Could you check a few things on this model? Use its own coordinates, in mm. Give positions to 0.01 mm unless a question says otherwise; leave off trailing zeros. Write each question's results on one line, items separated by ' | '. Start each with the question number.
Q1. Will this pin go through, and if not, where does the flat tip stop? P1, Ø1.5, axis at y = -1, z = -189, coming from the +X side.
Q2. If I drill on line 1 along X through (y, z) = (0.6, -190); line 2 along Z through (x, y) = (130, -0.45); line 3 along Z through (x, y) = (210, -0.75), over which ranges is the centre line in solid material (lowest first)?
Q3. If we section it at A-A, the plane y = 0.75: Give the number of separate pieces and of enclosed holes in the cut face, plus the area to 3 significant figures.
from build123d import *

# Parameters (mm, degrees)
SKETCH1_W               = 440
SKETCH1_H               = 400
BOSS_EXTRUDE1_DEPTH     = 2.5
SKETCH2_W               = 22
SKETCH2_H               = 22
CUT_EXTRUDE1_DEPTH      = 5
SKETCH3_R               = 2.6
CUT_EXTRUDE2_DEPTH      = 5
MIRROR2_COPY_1_SKETCH_W = 22
MIRROR2_COPY_1_SKETCH_H = 22
MIRROR2_COPY_1_DEPTH    = 5
MIRROR2_COPY_2_SKETCH_R = 2.6
MIRROR2_COPY_2_DEPTH    = 5
FILLET1_R               = 5
SKETCH4_W               = 25
SKETCH4_H               = 5
CUT_EXTRUDE3_DEPTH      = 5
LPATTERN1_COUNT         = 8
LPATTERN1_PITCH         = 55
SKETCH5_R               = 2.6
CUT_EXTRUDE4_DEPTH      = 5
LPATTERN2_COUNT         = 7
LPATTERN2_PITCH         = 55
SKETCH6_W               = 42.3
SKETCH6_H               = 42.3
CUT_EXTRUDE5_DEPTH      = 5
FILLET2_R               = 4
SKETCH7_R               = 2.6
CUT_EXTRUDE7_DEPTH      = 5
LPATTERN3_COUNT         = 2
LPATTERN3_PITCH         = 60
LPATTERN3_COUNT_DIR2    = 2
LPATTERN3_PITCH_DIR2    = 30
SKETCH8_R               = 4
SKETCH8_R_2             = 2.6
CUT_EXTRUDE8_DEPTH      = 5
CUT_EXTRUDE9_DEPTH      = 5


with BuildPart() as part:
    # Sketch1 → Boss-Extrude1 (new, symmetric)
    with BuildSketch(Plane(origin=(0, 0, 0), x_dir=(1, 0, 0), z_dir=(0, 1, 0))):
        Rectangle(SKETCH1_W, SKETCH1_H)
    extrude(amount=BOSS_EXTRUDE1_DEPTH, both=True)

    # Sketch2 → Cut-Extrude1 (cut)
    with BuildSketch(Plane(origin=(0, 2.5, 0), x_dir=(1, 0, 0), z_dir=(0, 1, 0))):
        with Locations((209, 189)):
            Rectangle(SKETCH2_W, SKETCH2_H)
    cut_extrude1 = extrude(amount=-CUT_EXTRUDE1_DEPTH, mode=Mode.SUBTRACT)

    # Sketch3 → Cut-Extrude2 (cut)
    with BuildSketch(Plane(origin=(0, 2.5, 0), x_dir=(1, 0, 0), z_dir=(0, 1, 0))):
        with Locations(Location((190, 190, 0), (0, 0, 270))):
            Circle(SKETCH3_R)
        with Locations(Location((210, 170, 0), (0, 0, 270))):
            Circle(SKETCH3_R)
    cut_extrude2 = extrude(amount=-CUT_EXTRUDE2_DEPTH, mode=Mode.SUBTRACT)

    # Mirror1: Cut-Extrude1, Cut-Extrude2 across plane
    add(cut_extrude1.mirror(Plane(origin=(0, 0, 0), x_dir=(0, 0, 1), z_dir=(1, 0, 0))), mode=Mode.SUBTRACT)
    add(cut_extrude2.mirror(Plane(origin=(0, 0, 0), x_dir=(0, 0, 1), z_dir=(1, 0, 0))), mode=Mode.SUBTRACT)

    # Mirror2: Cut-Extrude1, Cut-Extrude2 across plane
    add(cut_extrude1.mirror(Plane.XY), mode=Mode.SUBTRACT)
    add(cut_extrude2.mirror(Plane.XY), mode=Mode.SUBTRACT)

    # Mirror2 copy 1 sketch → Mirror2 copy 1 (cut)
    with BuildSketch(Plane(origin=(0, 2.5, 0), x_dir=(-1, 0, 0), z_dir=(0, 1, 0))):
        with Locations((209, 189)):
            Rectangle(MIRROR2_COPY_1_SKETCH_W, MIRROR2_COPY_1_SKETCH_H)
    extrude(amount=-MIRROR2_COPY_1_DEPTH, mode=Mode.SUBTRACT)

    # Mirror2 copy 2 sketch → Mirror2 copy 2 (cut)
    with BuildSketch(Plane(origin=(0, 2.5, 0), x_dir=(-1, 0, 0), z_dir=(0, 1, 0))):
        with Locations(Location((190, 190, 0), (0, 0, 270))):
            Circle(MIRROR2_COPY_2_SKETCH_R)
        with Locations(Location((210, 170, 0), (0, 0, 270))):
            Circle(MIRROR2_COPY_2_SKETCH_R)
    extrude(amount=-MIRROR2_COPY_2_DEPTH, mode=Mode.SUBTRACT)

    # Fillet1
    fillet1_edges = [part.edges().sort_by_distance(p)[0] for p in [
        (220, 0, -178),
        (198, 0, -178),
        (198, 0, -200),
        (-198, 0, -178),
        (-198, 0, -200),
        (-220, 0, -178),
        (-220, 0, 178),
        (-198, 0, 178),
        (-198, 0, 200),
        (198, 0, 178),
        (198, 0, 200),
        (220, 0, 178),
    ]]
    fillet(fillet1_edges, radius=FILLET1_R)

    # Sketch4 → Cut-Extrude3 (cut)
    with BuildSketch(Plane(origin=(0, 2.5, 0), x_dir=(1, 0, 0), z_dir=(0, 1, 0))):
        with Locations((-192.5, 137.5)):
            Rectangle(SKETCH4_W, SKETCH4_H)
    cut_extrude3 = extrude(amount=-CUT_EXTRUDE3_DEPTH, mode=Mode.SUBTRACT)

    # LPattern1: Cut-Extrude3 ×8
    with Locations(*[(i * LPATTERN1_PITCH, 0, 0) for i in range(1, LPATTERN1_COUNT)]):
        add(cut_extrude3, mode=Mode.SUBTRACT)

    # Sketch5 → Cut-Extrude4 (cut)
    with BuildSketch(Plane(origin=(0, 2.5, 0), x_dir=(1, 0, 0), z_dir=(0, 1, 0))):
        with Locations(Location((-165, 137.5, 0), (0, 0, 270))):
            Circle(SKETCH5_R)
    cut_extrude4 = extrude(amount=-CUT_EXTRUDE4_DEPTH, mode=Mode.SUBTRACT)

    # LPattern2: Cut-Extrude4 ×7
    with Locations(*[(i * LPATTERN2_PITCH, 0, 0) for i in range(1, LPATTERN2_COUNT)]):
        add(cut_extrude4, mode=Mode.SUBTRACT)

    # Sketch6 → Cut-Extrude5 (cut)
    with BuildSketch(Plane(origin=(0, 2.5, 0), x_dir=(1, 0, 0), z_dir=(0, 1, 0))):
        with Locations((0, 105)):
            Rectangle(SKETCH6_W, SKETCH6_H)
    extrude(amount=-CUT_EXTRUDE5_DEPTH, mode=Mode.SUBTRACT)

    # Fillet2
    fillet2_edges = [part.edges().sort_by_distance(p)[0] for p in [
        (21.15, 0, -126.15),
        (21.15, 0, -83.85),
        (-21.15, 0, -83.85),
        (-21.15, 0, -126.15),
    ]]
    fillet(fillet2_edges, radius=FILLET2_R)

    # Sketch7 → Cut-Extrude7 (cut)
    with BuildSketch(Plane(origin=(0, 2.5, 0), x_dir=(1, 0, 0), z_dir=(0, 1, 0))):
        with Locations(Location((30, 120, 0), (0, 0, 270))):
            Circle(SKETCH7_R)
    cut_extrude7 = extrude(amount=-CUT_EXTRUDE7_DEPTH, mode=Mode.SUBTRACT)

    # LPattern3: Cut-Extrude7 2 × 2
    with Locations(*[(-i * LPATTERN3_PITCH, 0, j * LPATTERN3_PITCH_DIR2) for i in range(LPATTERN3_COUNT) for j in range(LPATTERN3_COUNT_DIR2) if (i, j) != (0, 0)]):
        add(cut_extrude7, mode=Mode.SUBTRACT)

    # Sketch8 → Cut-Extrude8 (cut)
    with BuildSketch(Plane(origin=(0, 2.5, 0), x_dir=(1, 0, 0), z_dir=(0, 1, 0))):
        with Locations(Location((-115, 105, 0), (0, 0, 270))):
            Circle(SKETCH8_R)
        with Locations(Location((-100, 105, 0), (0, 0, 270))):
            Circle(SKETCH8_R_2)
        with Locations(Location((-130, 105, 0), (0, 0, 270))):
            Circle(SKETCH8_R_2)
    cut_extrude8 = extrude(amount=-CUT_EXTRUDE8_DEPTH, mode=Mode.SUBTRACT)

    # Mirror3: Cut-Extrude8 across plane
    add(cut_extrude8.mirror(Plane(origin=(0, 0, 0), x_dir=(0, 0, 1), z_dir=(1, 0, 0))), mode=Mode.SUBTRACT)

    # Sketch9 → Cut-Extrude9 (cut)
    with BuildSketch(Plane(origin=(0, 2.5, 0), x_dir=(1, 0, 0), z_dir=(0, 1, 0))):
        with BuildLine():
            Line((50, 175), (80, 175))
            ThreePointArc((80, 175), (90, 165), (80, 155))
            Line((80, 155), (50, 155))
            ThreePointArc((50, 155), (40, 165), (50, 175))
        make_face()
    cut_extrude9 = extrude(amount=-CUT_EXTRUDE9_DEPTH, mode=Mode.SUBTRACT)

    # Mirror4: Cut-Extrude9 across plane
    add(cut_extrude9.mirror(Plane(origin=(0, 0, 0), x_dir=(0, 0, 1), z_dir=(1, 0, 0))), mode=Mode.SUBTRACT)


solid = part.part
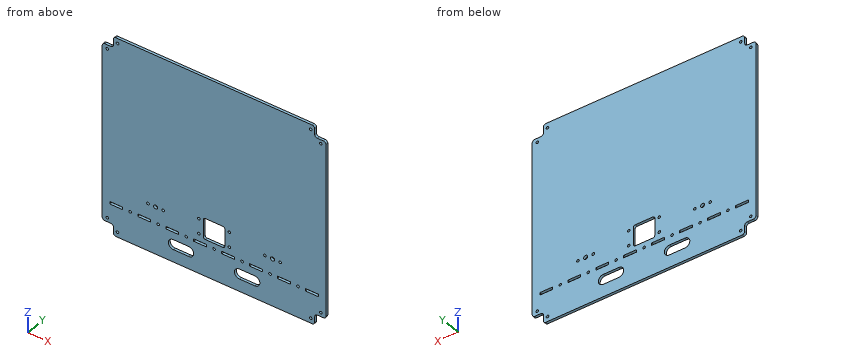
Final values:
1) P1: stops at x = 198
2) line 1: x = -198 to -192.6, -187.4 to 187.4, 192.6 to 198 | line 2: z = -200 to -140, -135 to -107.6, -102.4 to 200 | line 3: z = -178 to -172.6, -167.4 to 167.4, 172.6 to 178
3) separate pieces: 1 | enclosed holes: 36 | area: 169,000 mm²
